```python
from build123d import *

# Parameters (mm, degrees)
FILLET1_R               = 1.524
CHAMFER1_SIZE           = 0.762
CUT_EXTRUDE1_DEPTH      = 41.411152639
CUT_EXTRUDE1_DEPTH_BACK = 41.411152639
SKETCH3_RX              = 6.8453
SKETCH3_RY              = 1.2192


with BuildPart() as part:
    # Sketch2 → Revolve1 (revolve)
    with BuildSketch(Plane.XY, mode=Mode.PRIVATE) as revolve1_sk:
        with BuildLine():
            Line((0, 0), (-9.525, 0))
            Line((-9.525, 0), (-9.525, 3.175))
            Line((-9.525, 3.175), (-8.001, 3.175))
            Line((-8.001, 3.175), (-8.001, 4.699))
            Line((-8.001, 4.699), (-6.477, 4.699))
            Line((-6.477, 4.699), (-4.0386, 21.5392))
            ThreePointArc((-4.0386, 21.5392), (-4.775092358, 22.313794174), (-4.01298473, 23.0632))
            Line((-4.01298473, 23.0632), (-3.1496, 23.0632))
            ThreePointArc((-3.1496, 23.0632), (-5.385123327, 31.379708264), (0, 38.1))
            Line((0, 38.1), (0, 0))
        make_face()
    revolve(revolve1_sk.sketch.rotate(Axis((0, 0, 0), (0, 1, 0)), 270), axis=Axis((0, 0, 0), (0, 1, 0)))

    # Fillet1
    fillet1_edges = [part.edges().sort_by_distance(p)[0] for p in [
        (0, 4.699, 8.001),
    ]]
    fillet(fillet1_edges, radius=FILLET1_R - 0.0001)  # a hair under: the kernel refuses the full size

    # Chamfer1
    chamfer1_edges = [part.edges().sort_by_distance(p)[0] for p in [
        (0, 3.175, 9.525),
    ]]
    chamfer(chamfer1_edges, length=CHAMFER1_SIZE)

    # Sketch3 → Cut-Extrude1 (cut, two sides: drawn at the far end of the back side and taken through both)
    with BuildSketch(Plane.XY.offset(-CUT_EXTRUDE1_DEPTH_BACK)):
        with Locations(Location((3.136027313, 35.805849793), (0, 0, 65.87786559))):
            Ellipse(SKETCH3_RX, SKETCH3_RY)
    extrude(amount=CUT_EXTRUDE1_DEPTH + CUT_EXTRUDE1_DEPTH_BACK, mode=Mode.SUBTRACT)

    # Sketch4 → Revolve2 (revolve)
    with BuildSketch(Plane.XY, mode=Mode.PRIVATE) as revolve2_sk:
        with BuildLine():
            Line((0, 36.392009835), (0, 24.08140533))
            Line((0, 24.08140533), (-2.015653835, 24.08140533))
            ThreePointArc((-2.015653835, 24.08140533), (-3.958298201, 30.719797487), (0, 36.392009835))
        make_face()
    revolve(revolve2_sk.sketch.rotate(Axis((0, 38.1, 0), (0, -1, 0)), 90), axis=Axis((0, 38.1, 0), (0, -1, 0)))


solid = part.part
```
Source: CAD feature listing. Evaluate the final solid. Frame: model axes, mm. A direction names the side the tool comes from. Coordinates: 2 decimals unless noted, no trailing zeros. Write each loop counter-clockwise with the first axis right and the second up, starting at its lowest first coordinate (ties: lowest second). Pieces come first, ordered by that corner, then holes. Notation, with made-up numbers: (75, -25) -> (99, -25) arc R34 cw to (99, 13) -> close; hole circle Ø1 at (-20.5, 48.25). An arc over 180 degrees is marked (long way). Return JSON: item names as keys, results as strings. Group by question number.
1) Section query A-A, the plane y = 4. Return loops of the section in (x, z), plus the area to 3 significant figures.
2) Contact query for flat-ended pins moving along their axis: P1, Ø4, axis at x = -6.5, y = 27.5, coming from the +Z side; P2, Ø3, axis at x = 1, y = 25.5, coming from the -Z side; P3, Ø4, axis at x = -5, y = 30.5, coming from the -Z side. Output: stop coordinate, or through.
3) Ray query, line 1 along Y through (x, z) = (5.75, -6.5) (3 decimals); line 2 along Y through (x, z) = (-0.5, 7.75); line 3 along Z through (x, y) = (-5, 10.5). Return the intervals inside material, ascending.
4) Set-up query: faces 4 (the face through (0, 0, 0)), 5 (the face through (3, 23.063, -2)). Return all of +Z, -Z, +X, -X, +Y, -Y with unobstructed straight access to the full face (end or side cutting, diameter ignored); none if empty.
5) Mould query, pull axis Y, two halves, no side actions, for faces 1 (the face through (5.796, 1.223, 7.559)), 2 (the face through (3, 3.175, -8)), 3 (the face through (3.19, 13.24, 4.16)). Classes: +Y half, -Y half, draft (parallel to the pull), parting line (faces both ways), or undercut.
From the geometry:
{
 "1": {"outline": "circle Ø15.52 at (0, 0)", "area": "189 mm²"},
 "2": {"P1": "z = 3.04", "P2": "z = -5.23", "P3": "z = -4.66"},
 "3": {"line 1": "0 to 3.175", "line 2": "0 to 3.99", "line 3": "-2.6 to 2.6"},
 "4": {"face 4": "+Z, -Z, +X, -X, -Y", "face 5": "none"},
 "5": {"face 1": "draft", "face 2": "+Y half", "face 3": "undercut"}
}
